Autodesk Inventor part; units mm, degrees
ref_plane "YZ Plane" through (0, 0, 0) normal (1, 0, 0) x (0, 1, 0)
ref_plane "XZ Plane" through (0, 0, 0) normal (0, 1, 0) x (-1, 0, 0)
ref_plane "XY Plane" through (0, 0, 0) normal (0, 0, 1) x (1, 0, 0)
sketch "Sketch1" plane through (0, 0, 0) normal (0, 0, 1) x (1, 0, 0)
  line L0 (0, 0) -> (50.5, 0)
  line L1 (50.5, 0) -> (50.5, 26.8)
  line L2 (50.5, 26.8) -> (0, 26.8)
  line L3 (0, 26.8) -> (0, 0)
  dimension "d0" = 50.5
  dimension "d1" = 26.8
extrude "Extrusion1" add sketch "Sketch1" along normal blind 1.6
sketch "Esquisse2" plane through (0, 0, 1.6) normal (0, 0, 1) x (1, 0, 0)
  line L0 (0, 0) -> (50.5, 0) construction
  line L1 (50.5, 0) -> (50.5, 26.8) construction
  line L2 (50.5, 26.8) -> (0, 26.8) construction
  line L3 (0, 26.8) -> (0, 0) construction
  line L4 (3.35, 24.9) -> (47.15, 24.9) construction
  line L5 (47.15, 24.9) -> (47.15, 1.9) construction
  line L6 (47.15, 1.9) -> (3.35, 1.9) construction
  line L7 (3.35, 1.9) -> (3.35, 24.9) construction
  line L8 (25.25, 26.8) -> (25.25, 0) construction
  line L9 (0, 13.4) -> (50.5, 13.4) construction
  dimension "d4" = 43.8
  dimension "d5" = 23
hole "Perçage1" at (3.35, 24.9, 1.6) at (3.35, 1.9, 1.6) at (47.15, 24.9, 1.6) at (47.15, 1.9, 1.6) direction (0, 0, -1) diameter 2 end through all
fillet "Congé1" radius 2 4 edges at (0, 26.8, 0.8) (50.5, 26.8, 0.8) (50.5, 0, 0.8) (0, 0, 0.8)
sketch "Esquisse3" plane through (0, 0, 1.6) normal (0, 0, 1) x (1, 0, 0)
  arc A0 (0, 2) -> (2, 0) centre (2, 2) ccw construction
  line L0 (2, 0) -> (48.5, 0) construction
  arc A1 (48.5, 0) -> (50.5, 2) centre (48.5, 2) ccw construction
  line L1 (50.5, 2) -> (50.5, 24.8) construction
  arc A2 (50.5, 24.8) -> (48.5, 26.8) centre (48.5, 24.8) ccw construction
  line L2 (48.5, 26.8) -> (2, 26.8) construction
  arc A3 (2, 26.8) -> (0, 24.8) centre (2, 24.8) ccw construction
  line L3 (0, 24.8) -> (0, 2) construction
  circle A4 centre (47.15, 24.9) radius 1 construction
  circle A5 centre (3.35, 24.9) radius 1 construction
  circle A6 centre (3.35, 1.9) radius 1 construction
  circle A7 centre (47.15, 1.9) radius 1 construction
  line L4 (0, 22.9) -> (50.5, 22.9)
  line L5 (50.5, 22.9) -> (50.5, 3.9)
  line L6 (50.5, 3.9) -> (0, 3.9)
  line L7 (0, 3.9) -> (0, 22.9)
  line L8 (25.25, 26.8) -> (25.25, 0) construction
  line L9 (0, 13.4) -> (50.5, 13.4) construction
  point P0 (0, 0)
  dimension "d14" = 19
extrude "Extrusion2" add sketch "Esquisse3" along normal blind 8
sketch "Esquisse4" plane through (0, 0, 0) normal (0, 0, -1) x (-1, 0, 0)
  circle A0 centre (-47.15, 24.9) radius 1 construction
  circle A1 centre (-3.35, 24.9) radius 1 construction
  circle A2 centre (-3.35, 1.9) radius 1 construction
  circle A3 centre (-47.15, 1.9) radius 1 construction
  arc A4 (-2, 0) -> (0, 2) centre (-2, 2) ccw construction
  line L0 (0, 24.8) -> (0, 2) construction
  arc A5 (0, 24.8) -> (-2, 26.8) centre (-2, 24.8) ccw construction
  line L1 (-48.5, 26.8) -> (-2, 26.8) construction
  arc A6 (-48.5, 26.8) -> (-50.5, 24.8) centre (-48.5, 24.8) ccw construction
  line L2 (-50.5, 2) -> (-50.5, 24.8) construction
  arc A7 (-50.5, 2) -> (-48.5, 0) centre (-48.5, 2) ccw construction
  line L3 (-2, 0) -> (-48.5, 0) construction
  line L4 (-34, 17.9) -> (-16, 17.9)
  line L5 (-16, 17.9) -> (-16, 8.9)
  line L6 (-16, 8.9) -> (-34, 8.9)
  line L7 (-34, 8.9) -> (-34, 17.9)
  line L8 (-50.5, 13.4) -> (0, 13.4) construction
  point P0 (0, 0)
  dimension "d17" = 18
  dimension "d18" = 9
  dimension "d19" = 16
extrude "Extrusion3" add sketch "Esquisse4" along normal blind 2.8
sketch "Esquisse5" plane through (0, 0, 0) normal (0, 0, -1) x (-1, 0, 0)
  line L0 (-16, 17.9) -> (-16, 8.9) construction
  line L1 (-16, 8.9) -> (-34, 8.9) construction
  line L2 (-34, 8.9) -> (-34, 17.9) construction
  line L3 (-34, 17.9) -> (-16, 17.9) construction
  circle A0 centre (-47.15, 24.9) radius 1 construction
  circle A1 centre (-3.35, 24.9) radius 1 construction
  circle A2 centre (-3.35, 1.9) radius 1 construction
  circle A3 centre (-47.15, 1.9) radius 1 construction
  arc A4 (-2, 0) -> (0, 2) centre (-2, 2) ccw construction
  line L4 (0, 24.8) -> (0, 2) construction
  arc A5 (0, 24.8) -> (-2, 26.8) centre (-2, 24.8) ccw construction
  line L5 (-48.5, 26.8) -> (-2, 26.8) construction
  arc A6 (-48.5, 26.8) -> (-50.5, 24.8) centre (-48.5, 24.8) ccw construction
  line L6 (-50.5, 2) -> (-50.5, 24.8) construction
  arc A7 (-50.5, 2) -> (-48.5, 0) centre (-48.5, 2) ccw construction
  line L7 (-2, 0) -> (-48.5, 0) construction
  line L8 (-44, 21.9) -> (-16, 21.9)
  line L9 (-16, 21.9) -> (-16, 4.9)
  line L10 (-16, 4.9) -> (-44, 4.9)
  line L11 (-44, 4.9) -> (-44, 21.9)
  line L12 (-16, 17.9) -> (-34, 17.9) construction
  line L13 (-34, 17.9) -> (-34, 8.9) construction
  line L14 (-34, 8.9) -> (-16, 8.9) construction
  line L15 (-16, 8.9) -> (-16, 17.9) construction
  line L16 (-50.5, 13.4) -> (0, 13.4) construction
  point P0 (0, 0)
  dimension "d22" = 28
  dimension "d23" = 17
extrude "Extrusion4" add sketch "Esquisse5" along normal blind 1
sketch "Esquisse6" plane through (0, 0, 1.6) normal (0, 0, 1) x (1, 0, 0)
  line L0 (0, 22.9) -> (50.5, 22.9) construction
  line L1 (50.5, 22.9) -> (50.5, 24.8) construction
  arc A0 (50.5, 24.8) -> (48.5, 26.8) centre (48.5, 24.8) ccw construction
  line L2 (48.5, 26.8) -> (2, 26.8) construction
  arc A1 (2, 26.8) -> (0, 24.8) centre (2, 24.8) ccw construction
  line L3 (0, 24.8) -> (0, 22.9) construction
  circle A2 centre (47.15, 24.9) radius 1 construction
  circle A3 centre (3.35, 24.9) radius 1 construction
  line L4 (21.25, 25) -> (29.25, 25) construction
  line L5 (50.5, 3.9) -> (0, 3.9) construction
  line L6 (0, 3.9) -> (0, 2) construction
  arc A4 (0, 2) -> (2, 0) centre (2, 2) ccw construction
  line L7 (2, 0) -> (48.5, 0) construction
  arc A5 (48.5, 0) -> (50.5, 2) centre (48.5, 2) ccw construction
  line L8 (50.5, 2) -> (50.5, 3.9) construction
  circle A6 centre (3.35, 1.9) radius 1 construction
  circle A7 centre (47.15, 1.9) radius 1 construction
  line L9 (25.25, 26.8) -> (25.25, 0) construction
  point P0 (0, 0)
  point P1 (26.5, 25)
  point P2 (24, 25)
  dimension "d26" = 8
  dimension "d27" = 1.8
  dimension "d28" = 2.5
hole "Perçage2" at (21.25, 25, 1.6) at (29.25, 25, 1.6) at (26.5, 25, 1.6) at (24, 25, 1.6) direction (0, 0, -1) diameter 0.8 end through all
sketch "Esquisse7" plane through (0, 0, 9.6) normal (0, 0, 1) x (1, 0, 0)
  line L0 (7.75, 18.4) -> (42.75, 18.4) construction
  line L1 (42.75, 18.4) -> (42.75, 8.4) construction
  line L2 (42.75, 8.4) -> (7.75, 8.4) construction
  line L3 (7.75, 8.4) -> (7.75, 18.4) construction
  line L4 (50.5, 22.9) -> (0, 22.9) construction
  line L5 (0, 22.9) -> (0, 3.9) construction
  line L6 (0, 3.9) -> (50.5, 3.9) construction
  line L7 (50.5, 3.9) -> (50.5, 22.9) construction
  line L8 (25.25, 22.9) -> (25.25, 3.9) construction
  line L9 (0, 13.4) -> (50.5, 13.4) construction
  point P0 (0, 0)
  dimension "d2" = 1.6
  dimension "d36" = 35
  dimension "d37" = 10
properties part number "C001"
Model file for the job. Use its own axes, mm. A direction names the side the tool comes from. Coordinates: 2 decimals unless noted, no trailing zeros. Order: outer loops, then holes, each group sorted by start corner. A loop starts at its lowest first (then second) coordinate and runs counter-clockwise, first axis right, second up. Notation, with made-up numbers: M -29,54.25 L -18,54.25 A37 cw -18,92.25 Z; hole C 23.25,31.5 d4. An arc over 180 degrees is marked long. Answer as CSV lines item,"result".
(1) Band-saw the part on C-C, the plane z = 8.5. List the corners of the cut face in (x, y).
Geometry says:
outline,"M 0,3.9 L 50.5,3.9 L 50.5,22.9 L 0,22.9 Z"
(2) Wall check: line 1 along Y through (x, z) = (47.15, 0.7); line 2 along Y through (x, z) = (24, 1.15); line 3 along X through (y, z) = (1.9, 1.05). Give the ranges that are in metal, low to high.
Geometry says:
line 1,"y = 0 to 0.9, 2.9 to 23.9, 25.9 to 26.8"
line 2,"y = 0 to 24.6, 25.4 to 26.8"
line 3,"x = 0 to 2.35, 4.35 to 46.15, 48.15 to 50.5"
(3) Band-saw the part on D-D, the plane x = 6. List the corners of the cut face in (y, z), then the cut area to 3 significant figures.
Geometry says:
outline,"M 0,0 L 26.8,0 L 26.8,1.6 L 22.9,1.6 L 22.9,9.6 L 3.9,9.6 L 3.9,1.6 L 0,1.6 Z"
area,"195 mm2"
(4) Pull direction Y, two halves, no side cores. Call faces 4 (the cylindrical face through (46.16, 25.03, 0.79)), 5 (the flat face through (50.5, 13, 5)), 6 (the flat face through (26, 3.9, 6)): +Y half, -Y half, draft (parallel to the pull), parting line (faces both ways), or undercut.
Geometry says:
face 4,"undercut"
face 5,"draft"
face 6,"-Y half"
(5) 3-axis set-ups, long thin cutter, end or side, ignore diameter. For faces 1 (the flat face through (44, 13.3, -0.5)), 2 (the flat face through (25, 8.9, -2)), 3 (the flat face through (25, 17.9, -2)): which of +Z, -Z, +X, -X, +Y, -Y reach the whole face in a straight line?
Geometry says:
face 1,"-Z, +X, +Y, -Y"
face 2,"-Z, +X, -X, -Y"
face 3,"-Z, +X, -X, +Y"
(6) Flat gauge pins, fed straight in: pin 1 (2.5 mm diameter, centred on x = 3.35, y = 24.9, fed in from -Z); pin 2 (1.4 mm diameter, centred on x = 29, z = -2, fed in from -Y); pin 3 (1.4 mm diameter, centred on x = 22, z = -1.5, fed in from +Y). Where does each tip first touch, or does it go through?
Geometry says:
pin 1,"stops at z = 0"
pin 2,"stops at y = 8.9"
pin 3,"stops at y = 21.9"
(7) Band-saw the part on A-A, the plane x = 47.15. List the corners of the cut face in (y, z), then the cut area to 3 significant figures.
Geometry says:
outline,"M 0,0 L 0.9,0 L 0.9,1.6 L 0,1.6 Z; M 2.9,0 L 23.9,0 L 23.9,1.6 L 22.9,1.6 L 22.9,9.6 L 3.9,9.6 L 3.9,1.6 L 2.9,1.6 Z; M 25.9,0 L 26.8,0 L 26.8,1.6 L 25.9,1.6 Z"
area,"188 mm2"
(8) Band-saw the part on B-B, the plane x = 17. List the corners of the cut face in (y, z).
Geometry says:
outline,"M 0,0 L 4.9,0 L 4.9,-1 L 8.9,-1 L 8.9,-2.8 L 17.9,-2.8 L 17.9,-1 L 21.9,-1 L 21.9,0 L 26.8,0 L 26.8,1.6 L 22.9,1.6 L 22.9,9.6 L 3.9,9.6 L 3.9,1.6 L 0,1.6 Z"
